from build123d import *

# Parameters (mm, degrees)
BASE_SKETCH_R      = 11.112881
FEATURE_A_DEPTH    = 9.525
FEATURE_B_SKETCH_W = 22.225762
FEATURE_B_SKETCH_H = 33.338516
FEATURE_B_DEPTH    = 5.09143
FILLET1_R          = 11.112754
FILLET2_R          = 11.112754
FEATURE_C_SKETCH_W = 88.7984
FEATURE_C_SKETCH_H = 23.139146
FEATURE_C_DEPTH    = 24.14143
FEATURE_D_SKETCH_W = 12.6492
FEATURE_D_SKETCH_H = 38.1
FEATURE_D_DEPTH    = 24.14143
FEATURE_E_SKETCH_W = 38.0492
FEATURE_E_SKETCH_H = 18.899378
FEATURE_E_DEPTH    = 24.14143


with BuildPart() as part:
    # Base Sketch → Feature A (new, symmetric)
    with BuildSketch(Plane.YZ):
        with Locations(Location((0, -22.225635, 0), (0, 0, 90))):
            Circle(BASE_SKETCH_R)
    extrude(amount=FEATURE_A_DEPTH, both=True)

    # Feature B Sketch → Feature B (add)
    with BuildSketch(Plane(origin=(-9.525, 0, 0), x_dir=(0, -1, 0), z_dir=(-1, 0, 0))):
        with Locations((0, -16.669258)):
            Rectangle(FEATURE_B_SKETCH_W, FEATURE_B_SKETCH_H)
    extrude(amount=FEATURE_B_DEPTH)

    # Fillet1
    fillet1_edges = [part.edges().sort_by_distance(p)[0] for p in [
        (-12.070715, 11.112881, -33.338516),
    ]]
    fillet(fillet1_edges, radius=FILLET1_R)

    # Fillet2
    fillet2_edges = [part.edges().sort_by_distance(p)[0] for p in [
        (-12.070715, -11.112881, -33.338516),
    ]]
    fillet(fillet2_edges, radius=FILLET2_R)

    # Feature C Sketch → Feature C (add)
    with BuildSketch(Plane.YZ.offset(9.525)):
        with Locations((0, 11.569573)):
            Rectangle(FEATURE_C_SKETCH_W, FEATURE_C_SKETCH_H)
    extrude(amount=-FEATURE_C_DEPTH)

    # Feature D Sketch → Feature D (add)
    with BuildSketch(Plane.YZ.offset(9.525)):
        with Locations((38.0746, 42.189146)):
            Rectangle(FEATURE_D_SKETCH_W, FEATURE_D_SKETCH_H)
        with Locations((-38.0746, 42.189146)):
            Rectangle(FEATURE_D_SKETCH_W, FEATURE_D_SKETCH_H)
    extrude(amount=-FEATURE_D_DEPTH)

    # Feature E Sketch → Feature E (add)
    with BuildSketch(Plane.YZ.offset(9.525)):
        with Locations((25.3746, 70.688835)):
            Rectangle(FEATURE_E_SKETCH_W, FEATURE_E_SKETCH_H)
        with Locations((-25.3746, 70.688835)):
            Rectangle(FEATURE_E_SKETCH_W, FEATURE_E_SKETCH_H)
    extrude(amount=-FEATURE_E_DEPTH)


solid = part.part
The model under review builds one solid part; all positions refer to its coordinate system, in mm. A direction names the side the tool comes from. Round coordinates to 2 decimals unless told otherwise and drop trailing zeros. Order: outer loops, then holes, each group sorted by start corner. A loop starts at its lowest first (then second) coordinate and runs counter-clockwise, first axis right, second up. Notation, with made-up numbers: (86, 7.5) -> (119, 7.5) arc R26 cw to (119, 36.5) -> close; hole circle Ø10 at (27.5, 60.5). An arc over 180 degrees is marked (long way). Write item = value, one per line. Start each with the question number.
Item 1: Consider section D-D on y = -34. Write out the cut boundary in (x, z) (3 decimals), plus the area to 3 significant figures.
Item 2: For line 1 along Y through (x, z) = (4.5, 59.5); line 2 along Z through (x, y) = (6.5, 27.5); line 3 along Y through (x, z) = (4.5, 74), list the stretches that pass through material, from the lowest coordinate up.
Item 3: Consider section B-B on x = 2.25. Write out the cut boundary in (y, z).
Item 4: Mouldability with a two-part tool opening along Z and no side actions: class faces 1 (the face through (-12.11, -7.77, -30.17)), 2 (the face through (-2, 19, 61.239)), 3 (the face through (-2, -6.35, 71)) as released by +Z, released by -Z, zero draft, split by the parting line, or undercut.
Item 5: For faces 4 (the face through (-2, 6.35, 71)), 5 (the face through (0.133, -0.489, -33.328)), 6 (the face through (-12, 11.113, -11)), 7 (the face through (-2, 31.75, 42)), list the 3-axis set-ups (+Z, -Z, +X, -X, +Y, -Y) from which the entire face can be reached by the end or side of a thin tool; tool diameter is ignored.
Item 6: Consider section C-C on y = 26. Write out the cut boundary in (x, z) (3 decimals), plus the area to 3 significant figures.
Item 7: Consider section A-A on z = 63.5. Write out the cut boundary in (x, y) (3 decimals).
Item 8: Clearance check with flat-ended pins moving along their axes: pin 1 Ø6 at (x, z) = (-11, -11.5) entering from -Y; pin 2 Ø4 at (x, z) = (-13, -8.5) entering from +Y; pin 3 Ø2 at (x, z) = (1, -2) entering from -Y. State where each tip first meets the part, or that it passes through.
Conclusion:
q1.outline = (-14.616, 0) -> (9.525, 0) -> (9.525, 80.139) -> (-14.616, 80.139) -> close
q1.area = 1,930 mm2
q2.line_1 = -44.4 to -31.75, 31.75 to 44.4
q2.line_2 = 0 to 23.14, 61.24 to 80.14
q2.line_3 = -44.4 to -6.35, 6.35 to 44.4
q3.outline = (-44.4, 0) -> (44.4, 0) -> (44.4, 80.14) -> (6.35, 80.14) -> (6.35, 61.24) -> (31.75, 61.24) -> (31.75, 23.14) -> (-31.75, 23.14) -> (-31.75, 61.24) -> (-6.35, 61.24) -> (-6.35, 80.14) -> (-44.4, 80.14) -> close; circle Ø22.23 at (0, -22.23)
q4.face_1 = released by -Z
q4.face_2 = undercut
q4.face_3 = zero draft
q5.face_4 = +Z, +X, -X
q5.face_5 = +X
q5.face_6 = -Z, +X, -X, +Y
q5.face_7 = +X, -X
q6.outline = (-14.616, 0) -> (9.525, 0) -> (9.525, 23.139) -> (-14.616, 23.139) -> close; (-14.616, 61.239) -> (9.525, 61.239) -> (9.525, 80.139) -> (-14.616, 80.139) -> close
q6.area = 1,010 mm2
q7.outline = (-14.616, -44.399) -> (9.525, -44.399) -> (9.525, -6.35) -> (-14.616, -6.35) -> close; (-14.616, 6.35) -> (9.525, 6.35) -> (9.525, 44.399) -> (-14.616, 44.399) -> close
q8.pin_1 = -11.11
q8.pin_2 = 11.11
q8.pin_3 = through
